CAD build for the part. Positions are in the model's coordinates, mm. A direction names the side the tool comes from. Coordinates: 2 decimals unless noted, no trailing zeros. Order: outer loops, then holes, each group sorted by start corner. A loop starts at its lowest first (then second) coordinate and runs counter-clockwise, first axis right, second up. Notation, with made-up numbers: M 34.25,6 L 73.25,6 A26 cw 73.25,20 Z; hole C -19.75,68 d8. An arc over 180 degrees is marked long. Write item = value, one per line.
from build123d import *

# Parameters (mm, degrees)
SKETCH1_W           = 400
SKETCH1_H           = 304.8
BOSS_EXTRUDE1_DEPTH = 482.6
SHELL1_T            = 20
CUT_EXTRUDE1_REACH  = 546.177
SKETCH2_R           = 15.904700308
SKETCH3_W           = 100
SKETCH3_H           = 130
CUT_EXTRUDE2_DEPTH  = 50
SKETCH4_W           = 60
SKETCH4_H           = 80
CUT_EXTRUDE3_DEPTH  = 30


with BuildPart() as part:
    # Sketch1 → Boss-Extrude1 (new body)
    with BuildSketch(Plane(origin=(0, 0, 0), x_dir=(1, 0, 0), z_dir=(0, 1, 0))):
        Rectangle(SKETCH1_W, SKETCH1_H)
    extrude(amount=BOSS_EXTRUDE1_DEPTH)

    # Shell1 (no face opened: a closed hollow body)
    add(offset(amount=-SHELL1_T, mode=Mode.PRIVATE), mode=Mode.SUBTRACT)

    # Sketch2 → Cut-Extrude1 (cut, up to next)
    with BuildSketch(Plane(origin=(0, 482.6, 0), x_dir=(1, 0, 0), z_dir=(0, 1, 0)), mode=Mode.PRIVATE) as cut_extrude1_sk1:
        with Locations(Location((106, 0, 0), (0, 0, 270))):
            Circle(SKETCH2_R)
    cut_extrude1_tool1 = extrude(cut_extrude1_sk1.sketch, amount=-CUT_EXTRUDE1_REACH, mode=Mode.PRIVATE) & part.part
    add(cut_extrude1_tool1.solids().sort_by_distance((106, 482.6, 0))[0], mode=Mode.SUBTRACT)

    # Sketch3 → Cut-Extrude2 (cut)
    with BuildSketch(Plane.XY.offset(152.4)):
        with Locations((-130, 397.6)):
            Rectangle(SKETCH3_W, SKETCH3_H)
    extrude(amount=-CUT_EXTRUDE2_DEPTH, mode=Mode.SUBTRACT)

    # Sketch4 → Cut-Extrude3 (cut)
    with BuildSketch(Plane.XZ):
        with Locations((-60, 0)):
            Rectangle(SKETCH4_W, SKETCH4_H)
    extrude(amount=-CUT_EXTRUDE3_DEPTH, mode=Mode.SUBTRACT)


solid = part.part
(1) Wall check: line 1 (X direction, y = 475.5, z = 0); line 2 (X direction, y = 260, z = -130.5); line 3 (Y direction, x = -177, z = 78). Give the ranges that are in metal, low to high. Write a range as from..to.
Evaluation:
line_1 = -200..90.1, 121.9..200
line_2 = -200..-180, 180..200
line_3 = 0..20, 462.6..482.6
(2) Slice it at A-A, the plane z = 0. Write the cut outline in (x, y).
Evaluation:
outline = M -200,0 L -90,0 L -90,20 L -180,20 L -180,462.6 L 90.1,462.6 L 90.1,482.6 L -200,482.6 Z; M -30,0 L 200,0 L 200,482.6 L 121.9,482.6 L 121.9,462.6 L 180,462.6 L 180,20 L -30,20 Z
(3) Pull direction Y, two halves, no side cores. Call faces 6 (the face through (180, 238, 2)), 7 (the face through (-131, 332.6, 143)), 8 (the face through (-3, 0, -2)), 9 (the face through (-90, 10, -1)): +Y half, -Y half, draft (parallel to the pull), parting line (faces both ways), or undercut.
Evaluation:
face_6 = undercut
face_7 = undercut
face_8 = -Y half
face_9 = draft
(4) Tool access for faces 1 (the face through (-80, 397, 143)), 2 (the face through (-60, 10, 40)), 3 (the face through (-3, 238, -132.4)), 4 (the face through (-3, 238, 152.4)), 5 (the face through (121.77, 472.74, -2.07)): list every direction of +Z, -Z, +X, -X, +Y, -Y with a clear straight run to the whole face (end or side of a thin tool).
Evaluation:
face_1 = +Z
face_2 = -Y
face_3 = none
face_4 = +Z, +X, -X, +Y, -Y
face_5 = +Y
(5) Pin check, flat tip, straight feed: pin 1 Ø6 at (x, z) = (-145, 108.5) entering from -Y. Stop position of the tip, or through.
Evaluation:
pin_1 = 0
(6) Slice it at B-B, the plane y = 66. Write the cut outline in (x, z), then the cut area to 3 significant figures.
Evaluation:
outline = M -200,-152.4 L 200,-152.4 L 200,152.4 L -200,152.4 Z; hole M -180,-132.4 L 180,-132.4 L 180,132.4 L -180,132.4 Z
area = 26,600 mm²
(7) Slice it at D-D, the plane z = -63.5. Write the cut outline in (x, y), then the cut area to 3 significant figures.
Evaluation:
outline = M -200,0 L 200,0 L 200,482.6 L -200,482.6 Z; hole M -180,20 L 180,20 L 180,462.6 L -180,462.6 Z
area = 33,700 mm²
(8) Slice it at C-C, the plane x = -101.5. Write the cut outline in (y, z).
Evaluation:
outline = M 0,-152.4 L 482.6,-152.4 L 482.6,152.4 L 462.6,152.4 L 462.6,-132.4 L 20,-132.4 L 20,132.4 L 332.6,132.4 L 332.6,152.4 L 0,152.4 Z
